Check sheet for the modelled part. Datum: model origin and axes. Units: mm. Face numbers are marked on the shaded views. A direction names the side the tool comes from. Coordinates: 2 decimals unless noted, no trailing zeros. Order: outer loops, then holes, each group sorted by start corner. A loop starts at its lowest first (then second) coordinate and runs counter-clockwise, first axis right, second up.
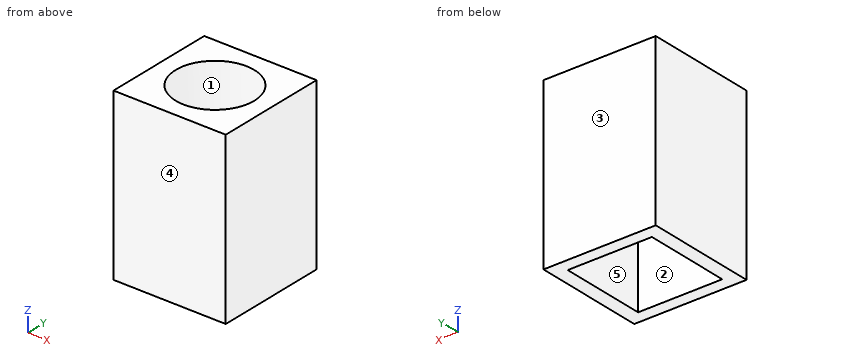
Solid Edge part; units mm, degrees
sketch "Sketch1" plane through (0, 0, 0) normal (0, 0, 1) x (1, 0, 0)
  line L0 (5, -5) -> (5, 5)
  line L1 (5, 5) -> (-5, 5)
  line L2 (-5, 5) -> (-5, -5)
  line L3 (-5, -5) -> (5, -5)
extrude "Protrusion1" add sketch "Sketch1" against normal blind 8
sketch "Sketch2" plane through (0, 0, 0) normal (0, 0, 1) x (1, 0, 0)
  circle A0 centre (0, 0) radius 3.5
extrude "ExtrudedCutout_1" cut sketch "Sketch2" along normal mid plane 71.7561
sketch "Sketch3" plane through (0, 0, -8) normal (0, 0, -1) x (1, 0, 0)
  line L0 (5, 5) -> (-5, 5)
  line L1 (-5, 5) -> (-5, -5)
  line L2 (-5, -5) -> (5, -5)
  line L3 (5, -5) -> (5, 5)
  line L4 (-3.7458, 3.875) -> (-3.7458, -3.875)
  line L5 (-3.7458, -3.875) -> (3.7458, -3.875)
  line L6 (3.7458, -3.875) -> (3.7458, 3.875)
  line L7 (3.7458, 3.875) -> (-3.7458, 3.875)
extrude "ExtrudedProtrusion_4" add sketch "Sketch3" along normal blind 7
sketch "Sketch4" plane through (0, 0, -8) normal (0, 0, -1) x (1, 0, 0)
  line L0 (3.7458, 3.875) -> (-3.7458, 3.875)
  line L1 (-3.7458, 3.875) -> (-3.7458, -3.875)
  line L2 (-3.7458, -3.875) -> (3.7458, -3.875)
  line L3 (3.7458, -3.875) -> (3.7458, 3.875)
extrude "Cutout1" cut sketch "Sketch4" along normal mid plane 8
(1) Thickness scan on probe 1 along X at (y, z) = (-1, -6); probe 2 along Y at (x, z) = (2, -6.75) (3 decimals); probe 3 along Y at (x, z) = (0, -0.85). Record the ranges inside material, lowest first.
Filled in:
probe 1: x = -5 to -3.75, 3.75 to 5
probe 2: y = -5 to -3.875, 3.875 to 5
probe 3: y = -5 to -3.5, 3.5 to 5
(2) Cross-section at D-D (z = -2.25). Enter the section's corners in (x, y).
Filled in:
outline: (-5, -5) - (5, -5) - (5, 5) - (-5, 5) - close; hole circle Ø7 at (0, 0)
(3) Cross-section at C-C (y = 0.75). Enter the section's corners in (x, z).
Filled in:
outline: (-5, -15) - (-3.75, -15) - (-3.75, -4) - (-3.42, -4) - (-3.42, 0) - (-5, 0) - close; (3.42, -4) - (3.75, -4) - (3.75, -15) - (5, -15) - (5, 0) - (3.42, 0) - close
(4) Tool access check on the marked faces 1 and 2. Record the directions out of +Z, -Z, +X, -X, +Y, -Y that give a thin tool (end or side, any length) a straight path to the whole face; none if there is none.
Filled in:
face 1: +Z, -Z
face 2: -Z
(5) Go/stop test with flat-tipped pins: P1, Ø5.5, axis at x = 0, y = 0, coming from the -Z side; P2, Ø3, axis at x = 1, y = -2, coming from the +Z side. Record where each tip stops, or that it passes through.
Filled in:
P1: passes through
P2: stops at z = 0
(6) Cross-section at A-A (z = -8.75). Enter the section's corners in (x, y) (3 decimals).
Filled in:
outline: (-5, -5) - (5, -5) - (5, 5) - (-5, 5) - close; hole (-3.746, -3.875) - (3.746, -3.875) - (3.746, 3.875) - (-3.746, 3.875) - close
(7) Release check for a two-part mould opening along Y. For the marked faces 3, 4 and 5 record: +Y half, -Y half, draft (parallel to the pull), parting line (faces both ways), or undercut.
Filled in:
face 3: +Y half
face 4: -Y half
face 5: undercut
(8) Cross-section at B-B (x = 0). Enter the section's corners in (y, z) (3 decimals), and give its area (4 significant figures).
Filled in:
outline: (-5, -15) - (-3.875, -15) - (-3.875, -4) - (-3.5, -4) - (-3.5, 0) - (-5, 0) - close; (3.5, -4) - (3.875, -4) - (3.875, -15) - (5, -15) - (5, 0) - (3.5, 0) - close
area: 36.75 mm2
